For this review, take the finished solid that the model builds, in its own axes (mm). Face numbers are marked on the shaded views. Coordinates: 2 decimals unless noted, no trailing zeros. Write each loop counter-clockwise with the first axis right and the second up, starting at its lowest first coordinate (ties: lowest second). Pieces come first, ordered by that corner, then holes. Notation, with made-up numbers: M -18,7.5 L 40,7.5 A16 ccw 40,26.5 Z; hole C 47.5,66 d7. An arc over 180 degrees is marked long. One line per question, with ' | ' between items.
from build123d import *

# Parameters (mm, degrees)
SKETCH002_R  = 30.035231
POCKET_DEPTH = 24
FILLET_R     = 3
FILLET001_R  = 3
FILLET002_R  = 1.5


with BuildPart() as part:
    # Sketch001 → Revolution (revolve)
    with BuildSketch(Plane.XZ):
        Polygon((-42.7, 0), (-42.7, 3.2), (-32.7, 3.2), (-32.7, 20.2), (0, 20.2), (0, 0), align=None)
    revolve(axis=Axis((0, 0, 0), (0, 0, 1)))

    # Sketch002 (on Face4 of Revolution) → Pocket (cut)
    with BuildSketch(Plane(origin=(0, 0, 20.2), x_dir=(-1, 0, 0), z_dir=(0, 0, 1))):
        Circle(SKETCH002_R)
    extrude(amount=-POCKET_DEPTH, mode=Mode.SUBTRACT)

    # Fillet
    fillet_edges = [part.edges().sort_by_distance(p)[0] for p in [
        (30.035231, 0, 0),
    ]]
    fillet(fillet_edges, radius=FILLET_R)

    # Fillet001
    fillet001_edges = [part.edges().sort_by_distance(p)[0] for p in [
        (42.7, 0, 0),
    ]]
    fillet(fillet001_edges, radius=FILLET001_R)

    # Fillet002
    fillet002_edges = [part.edges().sort_by_distance(p)[0] for p in [
        (32.7, 0, 20.2),
    ]]
    fillet(fillet002_edges, radius=FILLET002_R)


solid = part.part
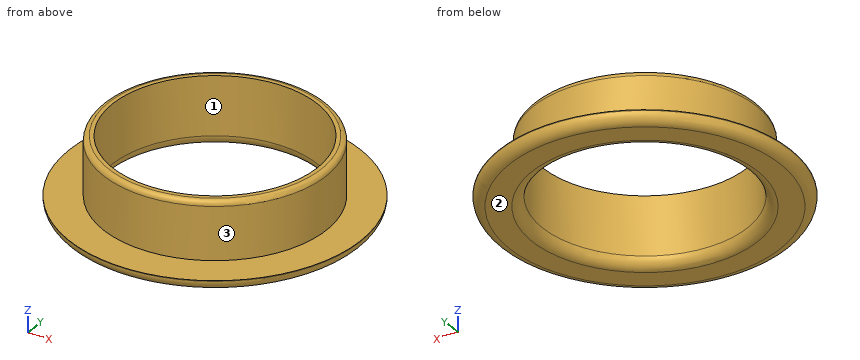
1) To check wall thickness, follow line 1 along Y through (x, z) = (0, 6.5); line 2 along X through (y, z) = (0.5, 4.5); line 3 along Z through (x, y) = (13, 35.5). State the ranges of each line that lie inside material, in increasing order. Write a range as [from, to].
Responses:
line 1: [-32.7, -30.04], [30.04, 32.7] | line 2: [-32.7, -30.03], [30.03, 32.7] | line 3: [0, 3.2]
2) Insertion check: pin 1 Ø8 at (y, z) = (-31, 4.5) entering from -X; pin 2 Ø1 at (y, z) = (-30, 3) entering from -X; pin 3 Ø8 at (x, z) = (14, 3.5) entering from -Y. Each pin has a flat end and moves straight along its axis. Give the tip position at first contact, or say it passes through.
Responses:
pin 1: x = -32.9 | pin 2: x = -30.87 | pin 3: y = -41.51
3) The part is to be moulded in two halves that separate along Y. For the marked faces 1, 2 and 3, say which applies: +Y half, -Y half, draft (parallel to the pull), parting line (faces both ways), or undercut.
Responses:
face 1: undercut | face 2: draft | face 3: parting line
4) We need section A-A on y = 0. State the section outline as (x, z) points.
Responses:
outline: M -42.7,3 A3 ccw -39.7,0 L -33.04,0 A3 ccw -30.04,3 L -30.04,20.2 L -31.2,20.2 A1.5 ccw -32.7,18.7 L -32.7,3.2 L -42.7,3.2 Z; M 30.04,3 A3 ccw 33.04,0 L 39.7,0 A3 ccw 42.7,3 L 42.7,3.2 L 32.7,3.2 L 32.7,18.7 A1.5 ccw 31.2,20.2 L 30.04,20.2 Z
5) We need section C-C on z = 4.25. State the section outline as (x, y) points.
Responses:
outline: C 0,0 d65.4; hole C 0,0 d60.07
